Can you work these out from the model? Positions are in its coordinate system, mm. A direction names the side the tool comes from. Coordinates: 2 decimals unless noted, no trailing zeros. Order: outer loops, then holes, each group sorted by start corner. A loop starts at its lowest first (then second) coordinate and runs counter-clockwise, first axis right, second up. Notation, with made-up numbers: (-33.75, 76.5) -> (-16.75, 76.5) arc R26 ccw to (-16.75, 94.5) -> close; hole circle Ø7 at (27, 23.5). An arc over 180 degrees is marked (long way). Answer in a Markdown table with one row per item.
Autodesk Fusion 360 part; units mm, degrees
sketch "Sketch1" plane through (0, 0, 0) normal (0, 0, 1) x (1, 0, 0)
  line L0 (-45, 8.5) -> (45, 8.5)
  line L1 (45, 8.5) -> (45, -8.5)
  line L2 (45, -8.5) -> (-45, -8.5)
  line L3 (-45, -8.5) -> (-45, 8.5)
  line L4 (-45, 8.5) -> (45, -8.5) construction
  line L5 (45, 8.5) -> (-45, -8.5) construction
  dimension "d1" = 90
  dimension "d2" = 17
extrude "Extrude1" add sketch "Sketch1" along normal blind 6
sketch "Sketch2" plane through (0, 0, 6) normal (0, 0, 1) x (-1, 0, 0)
  line L0 (45, 8.5) -> (-45, 8.5)
  line L1 (-45, 8.5) -> (-45, -8.5)
  line L2 (-45, -8.5) -> (45, -8.5)
  line L3 (45, -8.5) -> (45, 8.5)
  line L4 (45, -8.5) -> (39, -8.5) construction
  line L5 (39, -8.5) -> (39, -3.5) construction
  line L6 (39, -3.5) -> (45, -3.5) construction
  line L7 (45, -3.5) -> (45, -8.5) construction
  line L8 (-45, -8.5) -> (-39, -8.5) construction
  line L9 (-39, -8.5) -> (-39, -3.5) construction
  line L10 (-39, -3.5) -> (-45, -3.5) construction
  line L11 (-45, -3.5) -> (-45, -8.5) construction
  line L12 (45, -3.5) -> (39, -3.5)
  line L13 (39, -3.5) -> (39, 1.5)
  line L14 (39, 1.5) -> (45, 1.5)
  line L15 (45, 1.5) -> (45, -3.5)
  line L16 (-45, -3.5) -> (-39, -3.5)
  line L17 (-39, -3.5) -> (-39, 1.5)
  line L18 (-39, 1.5) -> (-45, 1.5)
  line L19 (-45, 1.5) -> (-45, -3.5)
  dimension "d5" = 6
  dimension "d6" = 5
  dimension "d7" = 6
  dimension "d8" = 5
  dimension "d9" = 5
  dimension "d10" = 5
extrude "Extrude2" cut sketch "Sketch2" against normal blind 9 contours L3 L12 L13 L14 L15 | L1 L16 L17 L18 L19
sketch "Sketch3" plane through (0, -8.5, 0) normal (0, -1, 0) x (1, 0, 0)
  line L0 (-45, 0) -> (45, 0)
  line L1 (45, 0) -> (45, 6)
  line L2 (45, 6) -> (-45, 6)
  line L3 (-45, 6) -> (-45, 0)
  line L4 (0, 6) -> (39, 6) construction
  line L5 (39, 0) -> (39, 6) construction
  line L6 (0, 6) -> (-39, 6) construction
  line L7 (-39, 6) -> (-39, 0) construction
  line L8 (0, 6) -> (0, 0)
  line L9 (0, 2.5249) -> (-20, 2.5249) construction
  line L10 (-20, 2.5249) -> (-20, 0) construction
  line L11 (0, 2.5249) -> (20, 2.5249) construction
  line L12 (-20, 0) -> (-25, 0)
  line L13 (-25, 0) -> (-25, 6)
  line L14 (-25, 6) -> (-20, 6)
  line L15 (-20, 6) -> (-20, 0)
  line L16 (20, 0) -> (25, 0)
  line L17 (25, 0) -> (25, 6)
  line L18 (25, 6) -> (20, 6)
  line L19 (20, 6) -> (20, 0)
extrude "Extrude3" add sketch "Sketch3" along normal blind 6 contours L0 L2 L12 L13 L14 L15 | L0 L2 L16 L17 L18 L19
sketch "Sketch4" plane through (-45, 0, 0) normal (-1, 0, 0) x (0, -1, 0)
  line L0 (-3.5, 0) -> (-3.5, 6)
  line L1 (-3.5, 6) -> (-8.5, 6)
  line L2 (-8.5, 6) -> (-8.5, 0)
  line L3 (-8.5, 0) -> (-3.5, 0)
  line L4 (-8.5, 6) -> (8.5, 6)
  line L5 (8.5, 6) -> (8.5, 0)
  line L6 (8.5, 0) -> (-8.5, 0)
  line L7 (-8.5, 0) -> (-8.5, 6)
  dimension "d15" = 17
  dimension "d16" = 6
extrude "Extrude4" add sketch "Sketch4" along normal blind 5
sketch "Sketch5" plane through (45, 0, 0) normal (1, 0, 0) x (0, 1, 0)
  line L0 (-1.5, 0) -> (-1.5, 6)
  line L1 (-1.5, 6) -> (-8.5, 6)
  line L2 (-8.5, 6) -> (-8.5, 0)
  line L3 (-8.5, 0) -> (-1.5, 0)
  line L4 (-8.5, 6) -> (8.5, 6)
  line L5 (8.5, 6) -> (8.5, 0)
  line L6 (8.5, 0) -> (-8.5, 0)
  line L7 (-8.5, 0) -> (-8.5, 6)
  dimension "d19" = 17
extrude "Extrude5" add sketch "Sketch5" along normal blind 5
(1) Suppose I cut it at C-C (z = 1.25). Please give me the cut outline in (x, y), and give its area (3 significant figures).
Response values:
| item | result |
|---|---|
| outline | (-50, -8.5) -> (-25, -8.5) -> (-25, -14.5) -> (-20, -14.5) -> (-20, -8.5) -> (20, -8.5) -> (20, -14.5) -> (25, -14.5) -> (25, -8.5) -> (50, -8.5) -> (50, 8.5) -> (-50, 8.5) -> close; hole (-45, -1.5) -> (-39, -1.5) -> (-39, 3.5) -> (-45, 3.5) -> close; hole (39, -1.5) -> (45, -1.5) -> (45, 3.5) -> (39, 3.5) -> close |
| area | 1,700 mm2 |
(2) We'd pull the mould along X, two halves only. Please class faces 5 (the flat face through (-42, -1.5, 3)), 6 (the flat face through (-50, 0, 3)), 7 (the flat face through (38, -8.5, 3)), 8 (the flat face through (-42, 3.5, 3)): +X half, -X half, draft (parallel to the pull), parting line (faces both ways), or undercut.
Response values:
| item | result |
|---|---|
| face 5 | undercut |
| face 6 | -X half |
| face 7 | draft |
| face 8 | undercut |
(3) I need wall thicknesses on line 1 (X direction, y = 1.75, z = 4.3); line 2 (Y direction, x = 42.5, z = 1.1); line 3 (X direction, y = -9.5, z = 4.2). Which ranges of each line are inside material? Lowest first, please. Write a range as [from, to].
Response values:
| item | result |
|---|---|
| line 1 | [-50, -45], [-39, 39], [45, 50] |
| line 2 | [-8.5, -1.5], [3.5, 8.5] |
| line 3 | [-25, -20], [20, 25] |
(4) Suppose I cut it at A-A (y = -11.75). Please give me the cut outline in (x, z).
Response values:
| item | result |
|---|---|
| outline | (-25, 0) -> (-20, 0) -> (-20, 6) -> (-25, 6) -> close; (20, 0) -> (25, 0) -> (25, 6) -> (20, 6) -> close |
(5) Suppose I cut it at B-B (x = 41.5). Please give me the cut outline in (y, z).
Response values:
| item | result |
|---|---|
| outline | (-8.5, 0) -> (-1.5, 0) -> (-1.5, 6) -> (-8.5, 6) -> close; (3.5, 0) -> (8.5, 0) -> (8.5, 6) -> (3.5, 6) -> close |
(6) Will these pins go through, and if not, where does the flat tip stop? pin 1 Ø3 at (y, z) = (-11, 3.5) entering from -X; pin 2 Ø1.8 at (y, z) = (-11, 1.5) entering from +X; pin 3 Ø1.8 at (x, z) = (-37, 2) entering from -Y; pin 4 Ø8 at (x, y) = (-11.5, 2) entering from -Z.
Response values:
| item | result |
|---|---|
| pin 1 | x = -25 |
| pin 2 | x = 25 |
| pin 3 | y = -8.5 |
| pin 4 | z = 0 |
(7) Suppose I cut it at D-D (y = 0.25). Please give me the cut outline in (x, z).
Response values:
| item | result |
|---|---|
| outline | (-50, 0) -> (-45, 0) -> (-45, 6) -> (-50, 6) -> close; (-39, 0) -> (39, 0) -> (39, 6) -> (-39, 6) -> close; (45, 0) -> (50, 0) -> (50, 6) -> (45, 6) -> close |
(8) On a 3-axis mill with a long thin cutter (end or side, diameter ignored), from which of +Z, -Z, +X, -X, +Y, -Y can I reach the whole of each face in a straight line? I mean faces 1 (the flat face through (-25, -11, 3)), 2 (the flat face through (25, -11, 3)), 3 (the flat face through (42, 3.5, 3)), 4 (the flat face through (20, -11, 3)). Say none if no direction works.
Response values:
| item | result |
|---|---|
| face 1 | +Z, -Z, -X, -Y |
| face 2 | +Z, -Z, +X, -Y |
| face 3 | +Z, -Z |
| face 4 | +Z, -Z, -Y |
